Geometry: final body of the model. Coordinates: model frame, mm. A direction names the side the tool comes from. Coordinates: 2 decimals unless noted, no trailing zeros. Order: outer loops, then holes, each group sorted by start corner. A loop starts at its lowest first (then second) coordinate and runs counter-clockwise, first axis right, second up. Notation, with made-up numbers: M 6.25,17 L 38.25,17 A12 cw 38.25,30 Z; hole C -18,70 d6. An arc over 180 degrees is marked long. Use CSV: the item, a comma, the result in double quotes. Start each with the question number.
Q1. Access query for faces 4 (the face through (0, 0, 0)), 5 (the face through (15.255, -19, -19)). Directions: +Z, -Z, +X, -X, +Y, -Y. A direction counts if a zero-diameter tool reaches every point of the face in a straight line with its end or side. Return the directions, or none.
Q2. Ray query, probe 1 along Y at (x, z) = (3.15, 0); probe 2 along X at (y, z) = (-8.5, -7); probe 3 along Y at (x, z) = (0.75, 12.5). Return the intervals inside material, ascending.
Q3. Section query A-A, the plane x = 2.5. Output: boundary loops of the cut face in (y, z).
Q4. First-contact query: P1, Ø2, axis at x = 13.5, y = -6, coming from the -Z side; P2, Ø8, axis at x = 1, y = 7, coming from the +Z side; P3, Ø17, axis at y = -6, z = 2, coming from the +X side. Flat tips, straight axial feed; report the tip coordinate or a pass-through.
Q5. Mould query, pull axis Z, two halves, no side actions, for faces 1 (the face through (6.507, -27.818, -6.177)), 2 (the face through (-2, 0, 0)), 3 (the face through (3.042, 14.334, 9.139)). Classes: +Z half, -Z half, draft (parallel to the pull), parting line (faces both ways), or undercut.
Q6. Section query B-B, the plane x = 12. Output: boundary loops of the cut face in (y, z), and give its area (3 significant figures).
from build123d import *


with BuildPart() as f1:
    # F0 (on Front) → F1 (revolve)
    with BuildSketch(Plane.XZ):
        with BuildLine():
            Line((7.6274327665, 20.4293505417), (13.3332152067, 25.8130880211))
            add(Edge.make_bspline(
                [(13.3332152067, 25.8130880211), (13.6873531533, 26.0396653478), (14.3178862388, 26.3941712558), (14.9677615599, 26.4891502818), (15.2545960447, 26.4951649422)],
                knots=[0.0753740232, 0.0753740232, 0.0753740232, 0.0753740232, 0.236653892, 0.3609439983, 0.3609439983, 0.3609439983, 0.3609439983], degree=3))
            Line((15.2545960447, 26.4951649422), (15.2545960447, 28.4951649422))
            Line((15.2545960447, 28.4951649422), (-2, 28.4951649422))
            Line((-2, 28.4951649422), (-2, 0))
            Line((-2, 0), (0, 0))
            Line((0, 0), (0, 17))
            Line((0, 17), (5.9999981131, 17))
            ThreePointArc((5.9999981131, 17), (6.7071048494, 17.292893174), (6.9999981131, 17.9999998731))
            Line((6.9999981131, 17.9999998731), (6.9999982367, 18.9746813235))
            ThreePointArc((6.9999982367, 18.9746813235), (7.1635437461, 19.7667886958), (7.6274327665, 20.4293505417))
        make_face()
    revolve(axis=Axis((-1, 0, 0), (-1, 0, 0)))


solid = f1.part
Responses:
1,face 4,"+X"
1,face 5,"+Z, -Z, +X, +Y, -Y"
2,probe 1,"y = -28.5 to -17, 17 to 28.5"
2,probe 2,"x = -2 to 0"
2,probe 3,"y = -25.61 to -11.52, 11.52 to 25.61"
3,outline,"C 0,0 d56.99; hole C 0,0 d34"
4,P1,"stops at z = -28.05"
4,P2,"stops at z = 28.34"
4,P3,"stops at x = 0"
5,face 1,"parting line"
5,face 2,"draft"
5,face 3,"undercut"
6,outline,"C 0,0 d56.99; hole C 0,0 d49.11"
6,area,"657 mm²"
